from build123d import *

# Parameters (mm, degrees)
SKETCH2_W          = 6.35
SKETCH2_H          = 50.8
CUT_EXTRUDE1_DEPTH = 6.35
SKETCH3_W          = 6.35
SKETCH3_H          = 38.1
CUT_EXTRUDE2_DEPTH = 6.35


with BuildPart() as part:
    # Sketch1 → Revolve1 (revolve)
    with BuildSketch(Plane(origin=(0, 0, 0), x_dir=(0, 0, -1), z_dir=(1, 0, 0)), mode=Mode.PRIVATE) as revolve1_sk:
        Polygon((0, 0), (0, 5.492242), (69.85, 5.492242), (69.85, 10.4529763), (95.25, 10.4529763), (95.25, 13.340207), (101.6, 13.340207), (101.6, 19.05), (158.75, 19.05), (158.75, 23.579455), (165.1, 23.579455), (165.1, 21.735161), (171.45, 21.735161), (171.45, 10.5689654), (203.2, 10.5689654), (203.2, 0), align=None)
    revolve(revolve1_sk.sketch.rotate(Axis((0, 0, 0), (0, 0, -1)), 90), axis=Axis((0, 0, 0), (0, 0, -1)))

    # Sketch2 → Cut-Extrude1 (cut)
    with BuildSketch(Plane(origin=(0, -5.492242, 0), x_dir=(-1, 0, 0), z_dir=(0, -1, 0))):
        with Locations((0, 25.4)):
            Rectangle(SKETCH2_W, SKETCH2_H)
    extrude(amount=-CUT_EXTRUDE1_DEPTH, mode=Mode.SUBTRACT)

    # Sketch3 → Cut-Extrude2 (cut)
    with BuildSketch(Plane(origin=(0, -19.05, 0), x_dir=(-1, 0, 0), z_dir=(0, -1, 0))):
        with Locations((0, 133.35)):
            Rectangle(SKETCH3_W, SKETCH3_H)
    extrude(amount=-CUT_EXTRUDE2_DEPTH, mode=Mode.SUBTRACT)


solid = part.part
Work out the finished part from the listing and answer in its coordinate system (mm). A direction names the side the tool comes from. Give positions to 0.01 mm unless a question says otherwise; leave off trailing zeros. Loops run counter-clockwise (first coordinate to the right, second up) from the corner with the lowest first, then second, coordinate; pieces in that order, holes last. Notation, with made-up numbers: (46, -16.5) - (70, -16.5) arc R23 cw to (70, 4.5) - close; hole circle Ø1 at (44.25, 47). An arc over 180 degrees is marked (long way). Answer in a Markdown table with one row per item.
(1) Section B-B (y = -8) is taken. Give the vertices of the cut face in (x, z).
Results list:
| item | result |
|---|---|
| outline | (-22.18, -165.1) - (-20.21, -165.1) - (-20.21, -171.45) - (-6.91, -171.45) - (-6.91, -203.2) - (6.91, -203.2) - (6.91, -171.45) - (20.21, -171.45) - (20.21, -165.1) - (22.18, -165.1) - (22.18, -158.75) - (17.29, -158.75) - (17.29, -101.6) - (10.68, -101.6) - (10.68, -95.25) - (6.73, -95.25) - (6.73, -69.85) - (-6.73, -69.85) - (-6.73, -95.25) - (-10.68, -95.25) - (-10.68, -101.6) - (-17.29, -101.6) - (-17.29, -158.75) - (-22.18, -158.75) - close |
(2) Section C-C (z = -133.5) is taken. Give the vertices of the cut face in (x, y) (3 decimals).
Results list:
| item | result |
|---|---|
| outline | (-3.175, -18.784) - (-3.175, -12.7) - (3.175, -12.7) - (3.175, -18.784) arc R19.05 ccw (long way) to start |
(3) Flat-ended cylindrical pins translate along their axes: pin 1 Ø4.5 at (y, z) = (-1, -28) entering from -X; pin 2 Ø3 at (x, y) = (0, -15) entering from -Z; pin 3 Ø1.5 at (x, z) = (-8, -166.5) entering from +Y. Find the tip coordinate at first contact, or state that the pin passes through.
Results list:
| item | result |
|---|---|
| pin 1 | stops at x = -5.49 |
| pin 2 | stops at z = -171.45 |
| pin 3 | stops at y = 20.49 |
(4) For a pull along X with two mould halves and no side action, classify faces 1 (the face through (8, 7, -95.25)), 2 (the face through (-2.83, -21.55, -168.32)), 3 (the face through (0, -2, -50.8)) as pulls with the +X half, pulls with the -X half, needs draft (parallel to the pull), parting line crosses it, or undercut.
Results list:
| item | result |
|---|---|
| face 1 | needs draft |
| face 2 | parting line crosses it |
| face 3 | undercut |
(5) Consider L1, parallel to Z at x = -3, y = -17; L2, parallel to Z at x = -16, y = -6.5; L3, parallel to Z at x = 2, y = 20. Determine where each line is inside the solid, lowest interval first. Write a range as [from, to].
Results list:
| item | result |
|---|---|
| L1 | z = [-171.45, -152.4], [-114.3, -101.6] |
| L2 | z = [-171.45, -101.6] |
| L3 | z = [-171.45, -158.75] |
(6) A tool of negligible diameter and unlimited length cuts with its end or side. For faces 4 (the face through (0, -16, -114.3)), 5 (the face through (-4.13, 18.597, -130.575)), 6 (the face through (7, 21, -165.1)), 7 (the face through (-3.175, -2, -25)), from which of +Z, -Z, +X, -X, +Y, -Y can it reach the whole face along a straight path? Write none if from no direction.
Results list:
| item | result |
|---|---|
| face 4 | -Y |
| face 5 | +Z |
| face 6 | -Z |
| face 7 | +Z, -Y |
